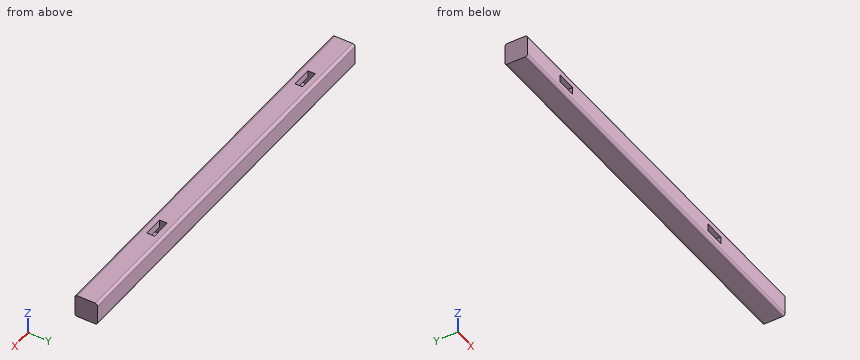
from build123d import *

# Parameters (mm, degrees)
F0_W      = 45
F0_H      = 45
F1_DEPTH  = 400
F2_R      = 5
F3_W      = 40
F3_H      = 15
F4_DEPTH  = 20
F5_W      = 40
F5_H      = 15
F6_DEPTH  = 20
F7_W      = 40
F7_H      = 15
F8_DEPTH  = 20
F9_W      = 40
F9_H      = 15
F10_DEPTH = 20


with BuildPart() as f1:
    # F0 (on Right) → F1 (new body, symmetric)
    with BuildSketch(Plane.YZ):
        Rectangle(F0_W, F0_H)
    extrude(amount=F1_DEPTH, both=True)

    # F2
    f2_edges = [f1.edges().sort_by_distance(p)[0] for p in [
        (0, -22.5, 22.5),
        (0, 22.5, 22.5),
        (0, -22.5, -22.5),
        (0, 22.5, -22.5),
    ]]
    fillet(f2_edges, radius=F2_R)

    # F3 (on face) → F4 (cut)
    with BuildSketch(Plane.XZ.offset(22.5)):
        with Locations((-280, 0)):
            Rectangle(F3_W, F3_H)
    extrude(amount=-F4_DEPTH, mode=Mode.SUBTRACT)

    # F5 (on face) → F6 (cut)
    with BuildSketch(Plane.XY.offset(22.5)):
        with Locations((-280, 0)):
            Rectangle(F5_W, F5_H)
    extrude(amount=-F6_DEPTH, mode=Mode.SUBTRACT)

    # F7 (on face) → F8 (cut)
    with BuildSketch(Plane.XY.offset(22.5)):
        with Locations((180, 0)):
            Rectangle(F7_W, F7_H)
    extrude(amount=-F8_DEPTH, mode=Mode.SUBTRACT)

    # F9 (on face) → F10 (cut)
    with BuildSketch(Plane.XZ.offset(22.5)):
        with Locations((180, 0)):
            Rectangle(F9_W, F9_H)
    extrude(amount=-F10_DEPTH, mode=Mode.SUBTRACT)


solid = f1.part
CAD build for the part. Positions are in the model's coordinates, mm. Coordinates: 2 decimals unless noted, no trailing zeros. Write each loop counter-clockwise with the first axis right and the second up, starting at its lowest first coordinate (ties: lowest second). Pieces come first, ordered by that corner, then holes. Notation, with made-up numbers: M 15,59.5 L 42,59.5 A23 ccw 42,78.5 Z; hole C 42.5,78 d10. An arc over 180 degrees is marked long. Return JSON: item names as keys, results as strings.
Item 1: Drop flat-ended pins along their axis: pin 1 Ø8 at (x, z) = (-277.5, -1.5) entering from -Y; pin 2 Ø5 at (x, y) = (-286.5, 3.5) entering from +Z. Give the stop position or say it passes through.
Findings below:
{"pin 1": "stops at y = -2.5", "pin 2": "stops at z = 2.5"}
Item 2: Slice it at A-A, the plane x = 185.5. Write the cut outline in (y, z).
Findings below:
{"outline": "M -22.5,-17.5 A5 ccw -17.5,-22.5 L 17.5,-22.5 A5 ccw 22.5,-17.5 L 22.5,17.5 A5 ccw 17.5,22.5 L 7.5,22.5 L 7.5,2.5 L -2.5,2.5 L -2.5,-7.5 L -22.5,-7.5 Z; M -22.5,7.5 L -7.5,7.5 L -7.5,22.5 L -17.5,22.5 A5 ccw -22.5,17.5 Z"}
Item 3: Probe line 1 (X direction, y = 3, z = 8); line 2 (Z direction, x = 8, y = 18); line 3 (Y direction, x = -297, z = 6.5). List the from-to ranges inside material, lowest first. Write a range as from..to.
Findings below:
{"line 1": "x = -400..-300, -260..160, 200..400", "line 2": "z = -22.47..22.47", "line 3": "y = 7.5..22.5"}
